Can you work these out from the drawing? Everything is in mm from the part's minimum corner. Coordinates: 2 decimals unless noted, no trailing zeros. Loops run counter-clockwise (first coordinate to the right, second up) from the corner with the lowest first, then second, coordinate; pieces in that order, holes last. Notation, with made-up numbers: M 51.25,48.25 L 94.25,48.25 A21 cw 94.25,74.25 Z; hole C 48.25,-37.5 d6. An arc over 180 degrees is marked long. Use CSV: the item, a comma, the result in double quotes. Start each with the question number.
Q1. If we section it at C-C (x = 10): Please give me the cut outline in (y, z).
Q2. If we section it at B-B (x = 49.5): Please give me the cut outline in (y, z), and give its area (3 significant figures).
Q3. If we section it at A-A (x = 30): Please give me the cut outline in (y, z), and give its area (3 significant figures).
Q4. Please list where these lines run through material, in increasing order: probe 1 along Y at (x, z) = (41.5, 1.6); probe 2 along Y at (x, z) = (30, 1.2); probe 3 along Y at (x, z) = (10.5, 2.35). Write a range as [from, to].
Q5. For pin 1 Ø5 at (x, y) = (30, 33.5) entering from -Z; pin 2 Ø1 at (x, z) = (19, 3) entering from +Y; pin 3 Ø1.5 at (x, z) = (2, 2) entering from -Y, each with a flat end and sliding along its axis, tell me the tip position at first contact or that it passes through.
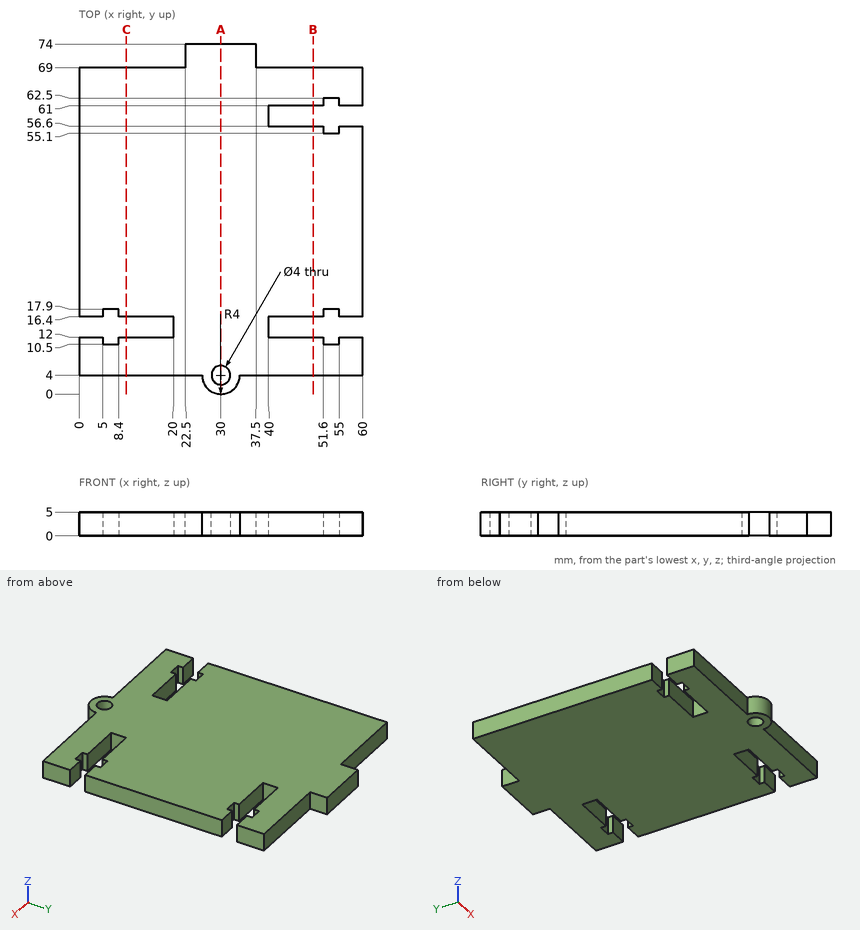
Results below:
1,outline,"M 4,0 L 12,0 L 12,5 L 4,5 Z; M 16.4,0 L 69,0 L 69,5 L 16.4,5 Z"
2,outline,"M 4,0 L 12,0 L 12,5 L 4,5 Z; M 16.4,0 L 56.6,0 L 56.6,5 L 16.4,5 Z; M 61,0 L 69,0 L 69,5 L 61,5 Z"
2,area,"281 mm^2"
3,outline,"M 0,0 L 2,0 L 2,5 L 0,5 Z; M 6,0 L 74,0 L 74,5 L 6,5 Z"
3,area,"350 mm^2"
4,probe 1,"[4, 12], [16.4, 56.6], [61, 69]"
4,probe 2,"[0, 2], [6, 74]"
4,probe 3,"[4, 12], [16.4, 69]"
5,pin 1,"z = 0"
5,pin 2,"y = 69"
5,pin 3,"y = 4"
